Read the model definition and answer for the solid it produces. Units are mm, in the model's axes. A direction names the side the tool comes from. Coordinates: 2 decimals unless noted, no trailing zeros. Loops run counter-clockwise (first coordinate to the right, second up) from the corner with the lowest first, then second, coordinate; pieces in that order, holes last. Notation, with made-up numbers: (54.5, -22.5) -> (72.5, -22.5) arc R36 ccw to (72.5, 14.5) -> close; hole circle Ø2 at (48.5, 40.5). An arc over 180 degrees is marked (long way). Answer as CSV lines item,"result".
```python
from build123d import *

# Parameters (mm, degrees)
CUT_EXTRUDE1_DEPTH      = 16
CUT_EXTRUDE1_DEPTH_BACK = 16


with BuildPart() as part:
    # Sketch1 → Revolve1 (revolve)
    with BuildSketch(Plane.XY):
        with BuildLine():
            Line((0, 0), (-15, 0))
            Line((-15, 0), (-15, 3))
            Line((-15, 3), (-13, 5))
            ThreePointArc((-13, 5), (-13.688325627, 10.216881481), (-10, 13.97))
            Line((-10, 13.97), (-10, 14.97))
            ThreePointArc((-10, 14.97), (-9.414213562, 16.384213562), (-8, 16.97))
            ThreePointArc((-8, 16.97), (-4.992249752, 32.435548835), (-7.5, 47.99))
            ThreePointArc((-7.5, 47.99), (-9.185787897, 49.659038605), (-8.5, 51.93))
            ThreePointArc((-8.5, 51.93), (-8.050914733, 62.26301618), (-2.5, 70.99))
            ThreePointArc((-2.5, 70.99), (-2.678187953, 73.885391492), (0, 75))
            Line((0, 75), (0, 70.99))
            Line((0, 70.99), (0, 51.93))
            Line((0, 51.93), (0, 47.99))
            Line((0, 47.99), (0, 16.97))
            Line((0, 16.97), (0, 14.97))
            Line((0, 14.97), (0, 13.97))
            Line((0, 13.97), (0, 5))
            Line((0, 5), (0, 3))
            Line((0, 3), (0, 0))
        make_face()
    revolve(axis=Axis((0, 0, 0), (0, 1, 0)))

    # Sketch2 → Cut-Extrude1 (cut, two sides)
    with BuildSketch(Plane.XY) as cut_extrude1_sk:
        Polygon((-4.249702272, 69.166839221), (-1.749702272, 64.836712202), (-3.048740377, 64.086712202), (-5.243895878, 67.888833061), (-5.823762224, 68.893191032), (-4.631125277, 69.887003162), align=None)
    extrude(amount=CUT_EXTRUDE1_DEPTH, mode=Mode.SUBTRACT)
    extrude(cut_extrude1_sk.sketch, amount=-CUT_EXTRUDE1_DEPTH_BACK, mode=Mode.SUBTRACT)


solid = part.part
```
Q1. A cutting plane is placed at B-B, the plane y = 10.5. Write down the section's boundary in (x, z).
Results:
outline,"circle Ø27.17 at (0, 0)"
Q2. Given pin 1 Ø1 at (x, z) = (-7.5, 8.5) entering from +Y; pin 2 Ø1 at (x, z) = (1.5, 10.5) entering from +Y; pin 3 Ø12 at (x, y) = (-4, 55.5) entering from -Z; pin 4 Ø8 at (x, z) = (-2, -10.5) entering from -Y, each flat-ended and moving along its own axis, determine where each tip first touches the part or whether it passes through.
Results:
pin 1,"stops at y = 13.6"
pin 2,"stops at y = 13.93"
pin 3,"stops at z = -9.21"
pin 4,"stops at y = 0"
Q3. Find the intervals of material crossed by probe 1 along Y at (x, z) = (9.75, 9); probe 2 along Y at (x, z) = (0.5, -1.75); probe 3 along Y at (x, z) = (-10, -1.75), in increasing order. Write a range as [from, to].
Results:
probe 1,"y = [0, 4.73], [5.45, 11.18]"
probe 2,"y = [0, 74.72]"
probe 3,"y = [0, 13.91]"
Q4. For a pull along Y with two mould halves and no side action, classify faces 3 (the face through (-3, 67, 0)), 4 (the face through (0, 0, 0)), 5 (the face through (14.985, 1.521, 0.66)) as pulls with the +Y half, pulls with the -Y half, needs draft (parallel to the pull), parting line crosses it, or undercut.
Results:
face 3,"undercut"
face 4,"pulls with the -Y half"
face 5,"needs draft"
Q5. A cutting plane is placed at A-A, the plane y = 45. Write down the section's boundary in (x, z), and give its area (3 significant figures).
Results:
outline,"circle Ø13.14 at (0, 0)"
area,"136 mm²"
Q6. For faces 1 (the face through (-3.89, 65.54, -0.09)), 2 (the face through (2.17, 14.48, -9.76)), determine the directions among +Z, -Z, +X, -X, +Y, -Y from which every point of the face is accessible in a straight line to the end or side of a thin tool.
Results:
face 1,"+Z, -Z"
face 2,"+Y"
